Can you work these out from the model? Positions are in its coordinate system, mm. Face numbers are marked on the shaded views. A direction names the side the tool comes from. Give positions to 0.01 mm unless a question says otherwise; leave off trailing zeros. Loops run counter-clockwise (first coordinate to the right, second up) from the corner with the lowest first, then second, coordinate; pieces in that order, holes last. Notation, with made-up numbers: M -35.75,-32 L 1.25,-32 A17 cw 1.25,-22 Z; hole C 5,-5.75 d4. An arc over 180 degrees is marked long. Use CSV: the item, a comma, the result in double quotes.
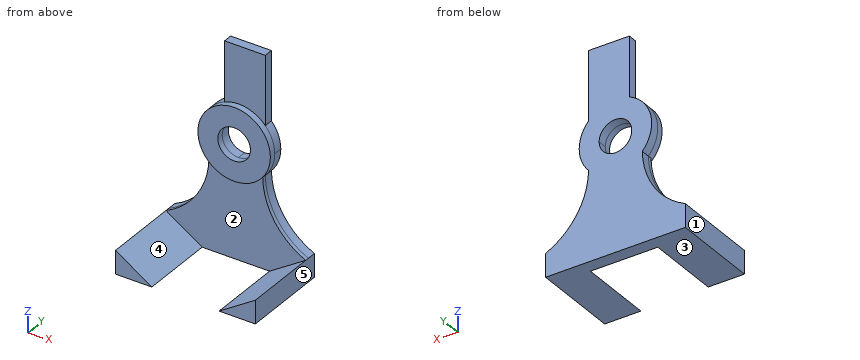
from build123d import *
from build123d import SkipClean  # not in build123d's __all__

# Parameters (mm, degrees)
F1_DEPTH = 5.55625
F2_R     = 22.225
F2_R_2   = 10.0000054
F3_DEPTH = 3.96875
F5_DEPTH = 2.38125
F7_DEPTH = 46.0375


# Not quite as in the source:
# - after a boolean that leaves OpenCascade's solid faulty, fix() repairs it


with BuildPart() as f1:
    # F0 (on Front) → F1 (new body)
    with BuildSketch(Plane.XZ):
        with BuildLine():
            ThreePointArc((8.5411146283, 90.3682841852), (21.9263912189, 91.5406597383), (33.5411154283, 84.7850490788))
            Line((33.5411154283, 84.7850490788), (33.5411154283, 127))
            Line((33.5411154283, 127), (8.5411146283, 127))
            Line((8.5411146283, 127), (8.5411146283, 90.3682841852))
        make_face()
        with BuildLine():
            ThreePointArc((17.0822292566, 47.625), (26.0827614415, 49.5290491023), (33.5411154283, 54.9149509212))
            Line((33.5411154283, 54.9149509212), (33.5411154283, 84.7850490788))
            ThreePointArc((33.5411154283, 84.7850490788), (21.9263912189, 91.5406597383), (8.5411146283, 90.3682841852))
            Line((8.5411146283, 90.3682841852), (8.5411146283, 75.050910392))
            ThreePointArc((8.5411146283, 75.050910392), (19.7830546485, 79.4783773401), (27.0822346566, 69.85))
            ThreePointArc((27.0822346566, 69.85), (24.1533008869, 62.7789283698), (17.0822292566, 59.8499946))
            Line((17.0822292566, 59.8499946), (17.0822292566, 47.625))
        make_face()
        with BuildLine():
            ThreePointArc((0.6233430849, 54.9149509212), (8.0816970717, 49.5290491023), (17.0822292566, 47.625))
            Line((17.0822292566, 47.625), (17.0822292566, 59.8499946))
            ThreePointArc((17.0822292566, 59.8499946), (8.3641663982, 64.9514810404), (8.5411146283, 75.050910392))
            Line((8.5411146283, 75.050910392), (8.5411146283, 90.3682841852))
            ThreePointArc((8.5411146283, 90.3682841852), (-4.6084304817, 74.6941619623), (0.6233430849, 54.9149509212))
        make_face()
        with BuildLine():
            Line((33.5411154283, 84.7850490788), (33.5411154283, 54.9149509212))
            ThreePointArc((33.5411154283, 54.9149509212), (37.8156487788, 61.8452551623), (39.3072292566, 69.85))
            ThreePointArc((39.3072292566, 69.85), (37.8156487788, 77.8547448377), (33.5411154283, 84.7850490788))
        make_face()
        with BuildLine():
            Line((17.0822292566, 0), (17.0822292566, 47.625))
            ThreePointArc((17.0822292566, 47.625), (8.0816970717, 49.5290491023), (0.6233430849, 54.9149509212))
            ThreePointArc((0.6233430849, 54.9149509212), (-6.7205760102, 30.7942081775), (-25.7802707434, 14.2875))
            Line((-25.7802707434, 14.2875), (-25.7802707434, 0))
            Line((-25.7802707434, 0), (17.0822292566, 0))
        make_face()
        with BuildLine():
            Line((33.5411154283, 0), (33.5411154283, 54.9149509212))
            ThreePointArc((33.5411154283, 54.9149509212), (26.0827614415, 49.5290491023), (17.0822292566, 47.625))
            Line((17.0822292566, 47.625), (17.0822292566, 0))
            Line((17.0822292566, 0), (33.5411154283, 0))
        make_face()
        with BuildLine():
            ThreePointArc((59.9447292566, 14.2875), (40.8850345234, 30.7942081775), (33.5411154283, 54.9149509212))
            Line((33.5411154283, 54.9149509212), (33.5411154283, 0))
            Line((33.5411154283, 0), (59.9447292566, 0))
            Line((59.9447292566, 0), (59.9447292566, 14.2875))
        make_face()
    extrude(amount=F1_DEPTH)

    # F2 (on face) → F3 (join)
    with BuildSketch(Plane.XZ.offset(5.55625)):
        with Locations((17.0822292566, 69.85)):
            Circle(F2_R)
        with Locations((17.0822292566, 69.85)):
            Circle(F2_R_2, mode=Mode.SUBTRACT)
    with SkipClean():  # cleaning this boolean's faces spoils the solid; the shape is the same uncleaned
        extrude(amount=F3_DEPTH)

    # F3_face (on face) + F4 (on face) → F5 (join)
    with BuildSketch(Plane(origin=(17.0822292566, -5.55625, 20.2916476737), x_dir=(1, 0, 0), z_dir=(0, -1, 0))):
        with BuildLine():
            ThreePointArc((16.4588861717, 34.6233032475), (0, 27.3333523263), (-16.4588861717, 34.6233032475))
            ThreePointArc((-16.4588861717, 34.6233032475), (-23.8028052668, 10.5025605039), (-42.8625, -6.0041476737))
            Line((-42.8625, -6.0041476737), (-42.8625, -20.2916476737))
            Line((-42.8625, -20.2916476737), (42.8625, -20.2916476737))
            Line((42.8625, -20.2916476737), (42.8625, -6.0041476737))
            ThreePointArc((42.8625, -6.0041476737), (23.8028052668, 10.5025605039), (16.4588861717, 34.6233032475))
        make_face()
    with BuildSketch(Plane.XZ.offset(5.55625)):
        with BuildLine():
            ThreePointArc((59.9447292566, 14.2875), (40.8850345234, 30.7942081775), (33.5411154283, 54.9149509212))
            ThreePointArc((33.5411154283, 54.9149509212), (17.0822292566, 47.625), (0.6233430849, 54.9149509212))
            ThreePointArc((0.6233430849, 54.9149509212), (-6.7205760102, 30.7942081775), (-25.7802707434, 14.2875))
            Line((-25.7802707434, 14.2875), (-25.7802707434, 0))
            Line((-25.7802707434, 0), (59.9447292566, 0))
            Line((59.9447292566, 0), (59.9447292566, 14.2875))
        make_face()
    extrude(amount=F5_DEPTH)

    add(f1.part.fix(), mode=Mode.REPLACE)

    # F6 (on face) → F7 (join)
    with BuildSketch(Plane.XZ.offset(7.9375)):
        Polygon((-25.7802707434, 14.2875), (-25.7802707434, 0), (-3.5552707434, 0), align=None)
        Polygon((59.9447292566, 14.2875), (37.7197292566, 0), (59.9447292566, 0), align=None)
    extrude(amount=F7_DEPTH)


solid = f1.part
Q1. I want a section at C-C, the plane z = 34.5. Please give me the cut outline in (x, y).
Model answer:
outline,"M -4.55,-7.94 L 38.72,-7.94 L 38.72,0 L -4.55,0 Z"
Q2. For the marked faces 1 and 2, which set-ups out of +Z, -Z, +X, -X, +Y, -Y let a thin tool reach every point of the face, with its end or its side?
Model answer:
face 1,"+Z, -Z, -X, +Y, -Y"
face 2,"-Y"
Q3. I want a section at D-D, the plane x = -15. Please give me the cut outline in (y, z) (1 decimal).
Model answer:
outline,"M -54,0 L 0,0 L 0,21.3 L -7.9,21.3 L -7.9,7.4 L -54,7.4 Z"
Q4. I want a section at A-A, the plane x = 25. Please give me the cut outline in (y, z) (1 decimal).
Model answer:
outline,"M -9.5,49.1 L -7.9,49.1 L -7.9,0 L 0,0 L 0,63.7 L -9.5,63.7 Z; M -9.5,76 L 0,76 L 0,127 L -5.6,127 L -5.6,90.6 L -9.5,90.6 Z"
Q5. I'm going to push flat-ended pins straight in: P1, Ø12, axis at x = 12, z = 51, coming from the -Y side (3 decimals); P2, Ø3, axis at y = -1.5, z = 102.5, coming from the +X side; P3, Ø1, axis at x = 2, z = 36.5, coming from the -Y side. Where does each tip first touch, or does it pass through?
Model answer:
P1,"y = -9.525"
P2,"x = 33.54"
P3,"y = -7.94"
Q6. Please list where these lines run through material, in increasing order: L1, parallel to X at y = -7.25, z = 69.85; L2, parallel to Y at x = 2.5, z = 73 (3 decimals); L3, parallel to Y at x = -7, z = 15. Write a range as from..to.
Model answer:
L1,"-5.14..7.08, 27.08..39.31"
L2,"-9.525..0"
L3,"-7.94..0"
Q7. If we mould it in two halves opening along X, with no side actions, what happens to the marked faces 3, 4 and 5? For each: released by +X, released by -X, zero draft, split by the parting line, or undercut.
Model answer:
face 3,"zero draft"
face 4,"undercut"
face 5,"released by +X"
Q8. I want a section at B-B, the plane y = -46.5. Please give me the cut outline in (x, z).
Model answer:
outline,"M -25.78,0 L -3.56,0 L -25.78,14.29 Z; M 37.72,0 L 59.94,0 L 59.94,14.29 Z"
